The listing builds one solid part. Answer for the finished solid, in the listing's coordinates (mm). Coordinates: 2 decimals unless noted, no trailing zeros. Write each loop counter-clockwise with the first axis right and the second up, starting at its lowest first coordinate (ties: lowest second). Pieces come first, ordered by that corner, then holes. Notation, with made-up numbers: M 85,85 L 90,85 A16 ccw 90,102 Z; hole C 73.25,1.5 d4. An arc over 180 degrees is marked long. Answer as CSV lines item,"result".
```python
from build123d import *

# Parameters (mm, degrees)
BOSS_EXTRUDE1_DEPTH = 3
FILLET1_R           = 5


with BuildPart() as part:
    # Sketch1 → Boss-Extrude1 (new body)
    with BuildSketch(Plane.XY):
        Polygon((0, 0), (56.5, 0), (56.5, 20), (10, 20), (10, 70), (-10, 70), (-10, 20), (-56.5, 20), (-56.5, 0), align=None)
        with BuildLine():
            Line((2.5, 62.5), (2.5, 27.5))
            ThreePointArc((2.5, 27.5), (0, 25), (-2.5, 27.5))
            Line((-2.5, 27.5), (-2.5, 62.5))
            ThreePointArc((-2.5, 62.5), (0, 65), (2.5, 62.5))
        make_face(mode=Mode.SUBTRACT)
        with BuildLine():
            Line((49, 7.5), (14, 7.5))
            ThreePointArc((14, 7.5), (11.5, 10), (14, 12.5))
            Line((14, 12.5), (49, 12.5))
            ThreePointArc((49, 12.5), (51.5, 10), (49, 7.5))
        make_face(mode=Mode.SUBTRACT)
        with BuildLine():
            Line((-49, 7.5), (-14, 7.5))
            ThreePointArc((-14, 7.5), (-11.5, 10), (-14, 12.5))
            Line((-14, 12.5), (-49, 12.5))
            ThreePointArc((-49, 12.5), (-51.5, 10), (-49, 7.5))
        make_face(mode=Mode.SUBTRACT)
    extrude(amount=BOSS_EXTRUDE1_DEPTH)

    # Fillet1
    fillet1_edges = [part.edges().sort_by_distance(p)[0] for p in [
        (-10, 70, 1.5),
        (10, 70, 1.5),
        (10, 20, 1.5),
        (56.5, 20, 1.5),
        (56.5, 0, 1.5),
        (-56.5, 0, 1.5),
        (-56.5, 20, 1.5),
        (-10, 20, 1.5),
    ]]
    fillet(fillet1_edges, radius=FILLET1_R)


solid = part.part
```
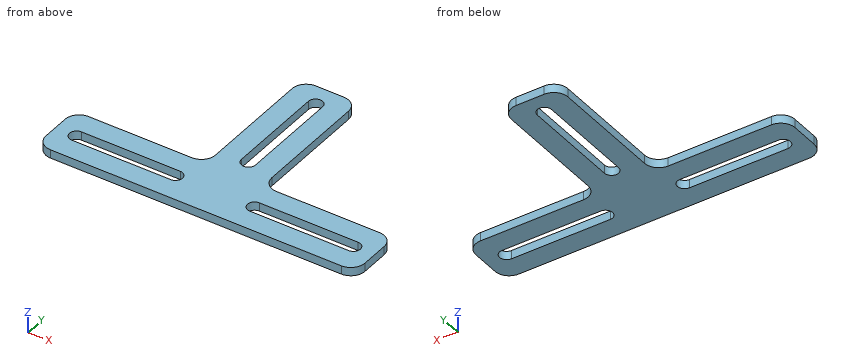
Q1. Find section B-B (z = 1.6). Give the vertices of the cut face in (x, y), and give its area (3 significant figures).
Output:
outline,"M -56.5,5 A5 ccw -51.5,0 L 51.5,0 A5 ccw 56.5,5 L 56.5,15 A5 ccw 51.5,20 L 15,20 A5 cw 10,25 L 10,65 A5 ccw 5,70 L -5,70 A5 ccw -10,65 L -10,25 A5 cw -15,20 L -51.5,20 A5 ccw -56.5,15 Z; hole M -49,7.5 L -14,7.5 A2.5 ccw -14,12.5 L -49,12.5 A2.5 ccw Z; hole M -2.5,27.5 A2.5 ccw 2.5,27.5 L 2.5,62.5 A2.5 ccw -2.5,62.5 Z; hole M 14,7.5 L 49,7.5 A2.5 ccw 49,12.5 L 14,12.5 A2.5 ccw Z"
area,"2,650 mm2"
Q2. Find section C-C (y = 53). Give the vertices of the cut face in (x, z).
Output:
outline,"M -10,0 L -2.5,0 L -2.5,3 L -10,3 Z; M 2.5,0 L 10,0 L 10,3 L 2.5,3 Z"
Q3. Find section A-A (x = -47). Give the vertices of the cut face in (y, z), and give its area (3 significant figures).
Output:
outline,"M 0,0 L 7.5,0 L 7.5,3 L 0,3 Z; M 12.5,0 L 20,0 L 20,3 L 12.5,3 Z"
area,"45.0 mm2"
Q4. A flat-ended cylindrical pin translates along its axis: pin 1 Ø0.9 at (x, z) = (-38, 1.5) entering from +Y. Find the tip coordinate at first contact, or state that the pin passes through.
Output:
pin 1,"y = 20"
Q5. Straight lines are drawn through the part: line 1 (X direction, y = 44, z = 2.7); line 2 (Y direction, x = -18, z = 2.4); line 3 (Y direction, x = 51, z = 0.15). For each, find the intervals that lie inside material, in ascending order.
Output:
line 1,"-10 to -2.5, 2.5 to 10"
line 2,"0 to 7.5, 12.5 to 20"
line 3,"0 to 8.5, 11.5 to 20"
